Check sheet for the modelled part. Datum: model origin and axes. Units: mm. Give positions to 0.01 mm unless a question says otherwise; leave off trailing zeros. Order: outer loops, then holes, each group sorted by start corner. A loop starts at its lowest first (then second) coordinate and runs counter-clockwise, first axis right, second up.
Item 1: Sectioned sample at C-C on y = -11. Record the boundary of the cut face in (x, z), and give its area (3 significant figures).
Item 2: Material ranges on line 1 along Z through (x, y) = (360, -7); line 2 along X through (y, z) = (-3.5, 122); line 3 along Z through (x, y) = (360, -16.9), recorded low to high.
Item 3: Gauge pin test, flat end, axial feed: P1, Ø15, axis at x = 46, z = 27, coming from the +Y side. Record the tip position at first contact, or that the pin passes through.
Item 4: Sectioned sample at A-A on x = 360. Record the boundary of the cut face in (y, z), and give its area (3 significant figures).
Item 5: Sectioned sample at B-B on z = 122. Record the boundary of the cut face in (x, y), and give its area (3 significant figures).
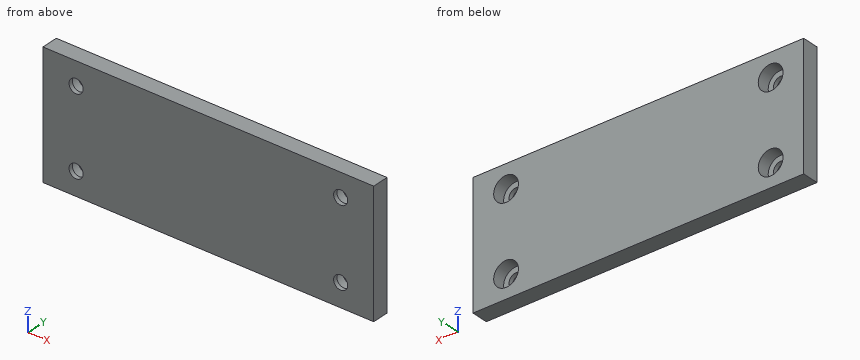
from build123d import *

# Parameters (mm, degrees)
F0_W           = 400
F0_H           = 150
F1_DEPTH       = 20
F2_D           = 17
F2_DEPTH       = 35
F2_CBORE_D     = 30
F2_CBORE_DEPTH = 15
F2_TIP         = 5.1073152617


with BuildPart() as f1:
    # F0 (on Front) → F1 (new body)
    with BuildSketch(Plane.XZ):
        with Locations((200, 75)):
            Rectangle(F0_W, F0_H)
    extrude(amount=F1_DEPTH)

    # F2
    with Locations(Plane(origin=(0, 0, 0), x_dir=(1, 0, 0), z_dir=(0, 1, 0))):
        with Locations((360, -122), (360, -28), (40, -122), (40, -28)):
            CounterBoreHole(F2_D / 2, F2_CBORE_D / 2, F2_CBORE_DEPTH, depth=F2_DEPTH)
            with Locations((0, 0, -(F2_DEPTH + F2_TIP / 2))):  # 118° drill point
                Cone(0, F2_D / 2, F2_TIP, mode=Mode.SUBTRACT)


solid = f1.part
Report:
1. outline: (0, 0) - (400, 0) - (400, 150) - (0, 150) - close; hole circle Ø30 at (40, 28); hole circle Ø30 at (40, 122); hole circle Ø30 at (360, 28); hole circle Ø30 at (360, 122)
1. area: 57,200 mm2
2. line 1: z = 0 to 13, 43 to 107, 137 to 150
2. line 2: x = 0 to 25, 55 to 345, 375 to 400
2. line 3: z = 0 to 19.5, 36.5 to 113.5, 130.5 to 150
3. P1: stops at y = -15
4. outline: (-20, 0) - (0, 0) - (0, 13) - (-15, 13) - (-15, 19.5) - (-20, 19.5) - close; (-20, 36.5) - (-15, 36.5) - (-15, 43) - (0, 43) - (0, 107) - (-15, 107) - (-15, 113.5) - (-20, 113.5) - close; (-20, 130.5) - (-15, 130.5) - (-15, 137) - (0, 137) - (0, 150) - (-20, 150) - close
4. area: 1,930 mm2
5. outline: (0, -20) - (31.5, -20) - (31.5, -15) - (25, -15) - (25, 0) - (0, 0) - close; (48.5, -20) - (351.5, -20) - (351.5, -15) - (345, -15) - (345, 0) - (55, 0) - (55, -15) - (48.5, -15) - close; (368.5, -20) - (400, -20) - (400, 0) - (375, 0) - (375, -15) - (368.5, -15) - close
5. area: 6,930 mm2
